The drawing under review shows one solid part. Ordinate dimensions are in mm from its lowest x, y, z. A direction names the side the tool comes from. Coordinates: 2 decimals unless noted, no trailing zeros. Order: outer loops, then holes, each group sorted by start corner. A loop starts at its lowest first (then second) coordinate and runs counter-clockwise, first axis right, second up.
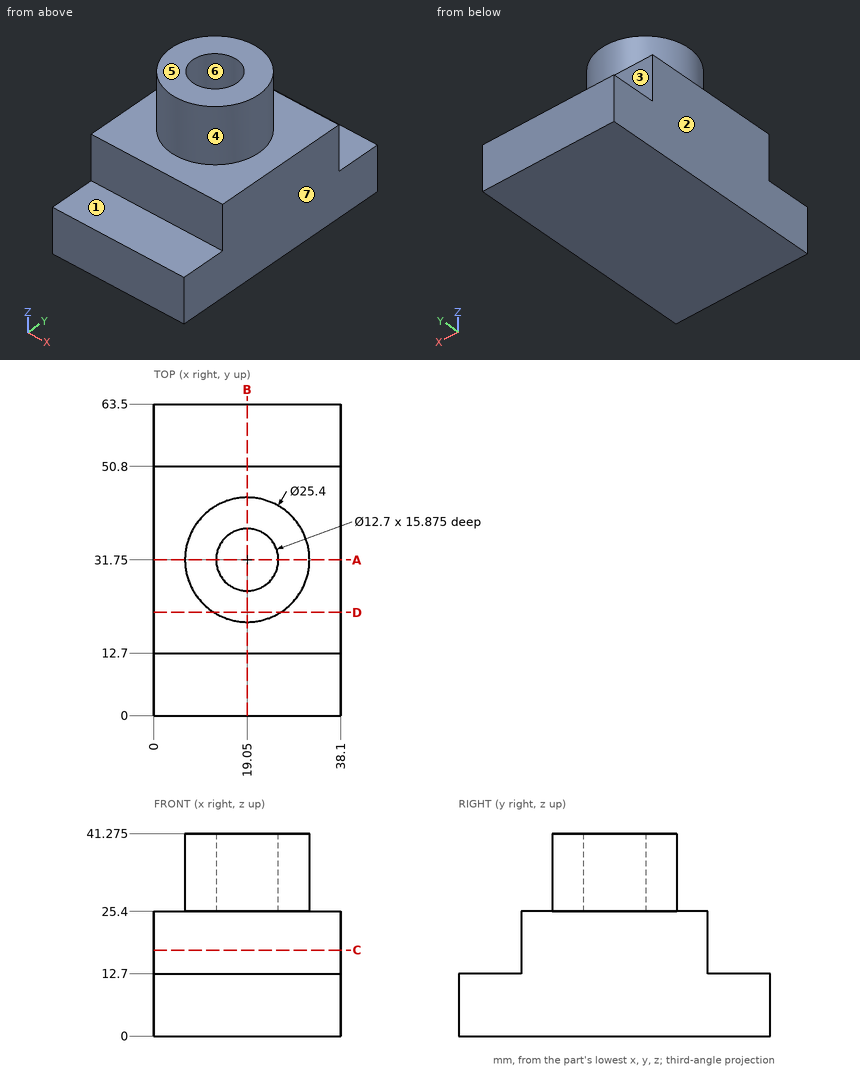
(1) Consider section B-B (x = 19.05). Give the boundary of the cut face in (y, z) (3 decimals).
(2) Tool access review of the marked faces 1, 2, 3 and 4: name each direction out of +Z, -Z, +X, -X, +Y, -Y from which nothing blocks a thin tool from reaching the whole face with its end or side.
(3) Consider section C-C (z = 17.5). Give the boundary of the cut face in (x, y), then the cut area to 3 significant figures.
(4) Wall thickness on line 1 (Y direction, x = 19.05, z = 38); line 2 (Z direction, x = 18, y = 18.5); line 3 (Y direction, x = 16, z = 25): over which ranges is each line inside the solid? List them lowest first.
(5) Consider section D-D (y = 21). Give the boundary of the cut face in (x, z) (3 decimals), then the cut area to 3 significant figures.
(6) Insertion check: pin 1 Ø6.5 at (x, z) = (27, 18) entering from +Y; pin 2 Ø6.5 at (x, y) = (25, 7) entering from +Z; pin 3 Ø6 at (x, y) = (33.5, 39.5) entering from +Z. Each pin has a flat end and moves straight along its axis. Give the tip position at first contact, or say it passes through.
(7) The part is to be moulded in two halves that separate along X. For the marked faces 5, 6 and 7, say which applies: +X half, -X half, draft (parallel to the pull), parting line (faces both ways), or undercut.
(8) Consider section A-A (y = 31.75). Give the boundary of the cut face in (x, z) (3 decimals), then the cut area to 3 significant figures.
Findings:
1. outline: (0, 0) - (63.5, 0) - (63.5, 12.7) - (50.8, 12.7) - (50.8, 25.4) - (44.45, 25.4) - (44.45, 41.275) - (38.1, 41.275) - (38.1, 25.4) - (25.4, 25.4) - (25.4, 41.275) - (19.05, 41.275) - (19.05, 25.4) - (12.7, 25.4) - (12.7, 12.7) - (0, 12.7) - close
2. face 1: +Z, +X, -X, -Y
2. face 2: +Z, -Z, -X, +Y, -Y
2. face 3: +Z, +X, -X, +Y
2. face 4: +Z
3. outline: (0, 12.7) - (38.1, 12.7) - (38.1, 50.8) - (0, 50.8) - close
3. area: 1,450 mm2
4. line 1: y = 19.05 to 25.4, 38.1 to 44.45
4. line 2: z = 0 to 25.4
4. line 3: y = 12.7 to 50.8
5. outline: (0, 0) - (38.1, 0) - (38.1, 25.4) - (25.812, 25.4) - (25.812, 41.275) - (12.288, 41.275) - (12.288, 25.4) - (0, 25.4) - close
5. area: 1,180 mm2
6. pin 1: stops at y = 50.8
6. pin 2: stops at z = 12.7
6. pin 3: stops at z = 25.4
7. face 5: draft
7. face 6: undercut
7. face 7: +X half
8. outline: (0, 0) - (38.1, 0) - (38.1, 25.4) - (31.75, 25.4) - (31.75, 41.275) - (25.4, 41.275) - (25.4, 25.4) - (12.7, 25.4) - (12.7, 41.275) - (6.35, 41.275) - (6.35, 25.4) - (0, 25.4) - close
8. area: 1,170 mm2
